Verification items for the finished model (mm, model axes). A direction names the side the tool comes from. Round coordinates to 2 decimals unless told otherwise and drop trailing zeros. Write each loop counter-clockwise with the first axis right and the second up, starting at its lowest first coordinate (ties: lowest second). Pieces come first, ordered by that corner, then holes. Notation, with made-up numbers: (-15.5, 2) - (38.5, 2) arc R35 ccw to (38.5, 37) - close; hole circle Ø8 at (-17.5, 78.25). An arc over 180 degrees is marked (long way). Answer as a JSON object with one key per item and string values. Group by question number.
1) Go/stop test with flat-tipped pins: pin 1 Ø2 at (x, z) = (-69, -39) entering from -Y; pin 2 Ø1.5 at (x, y) = (-13.5, 28.5) entering from -Z; pin 3 Ø4 at (x, y) = (-69.088, -30.988) entering from -Z. Record where each tip stops, or that it passes through.
2) Set-up check for faces 3 (the flat face through (1, 44.45, -47)), 4 (the cylindrical face through (-17.02, 21.68, 3.22)), 5 (the cylindrical face through (32.747, 47.669, -21.646)): record each of +Z, -Z, +X, -X, +Y, -Y from which the full face is reachable in a straight line by a thin tool's end or side.
3) Section check C-C (y = -1.5). Enter the section's corners in (x, z), then the cut area to 3 significant figures.
4) Section check A-A (x = 23.5). Enter the section's corners in (y, z) (3 decimals).
5) Mould release check, pull along Z, two halves, no side actions. Record for faces 1 (the cylindrical face through (32.747, 47.669, -59.746)), 2 (the cylindrical face through (66.568, 29.056, 3.131)): +Z half, -Z half, draft (parallel to the pull), parting line (faces both ways), or undercut.
6) Section check D-D (x = -75). Enter the section's corners in (y, z).
7) Section check B-B (z = -18.65). Enter the section's corners in (x, y) (3 decimals), then the cut area to 3 significant figures.
8) Thickness scan on line 1 (X direction, y = 48.75, z = -18.65) (3 decimals); line 2 (Y direction, x = -78, z = -62); line 3 (Z direction, x = 16, y = 22.5). Record the ranges inside material, lowest first.
```python
from build123d import *

# Parameters (mm, degrees)
SKETCH1_W           = 177.8
SKETCH1_H           = 101.6
SKETCH1_R           = 3.175
SKETCH1_W_2         = 46.99
SKETCH1_H_2         = 46.99
BOSS_EXTRUDE2_DEPTH = 6.35
SKETCH2_W           = 177.8
SKETCH2_H           = 6.35
BOSS_EXTRUDE3_DEPTH = 95.25
FILLET1_R           = 6.35
SKETCH3_R           = 4.065
CUT_EXTRUDE1_DEPTH  = 152.4


with BuildPart() as part:
    # Sketch1 → Boss-Extrude2 (new body)
    with BuildSketch(Plane.XY):
        Rectangle(SKETCH1_W, SKETCH1_H)
        with Locations((-69.088, 30.988)):
            Circle(SKETCH1_R, mode=Mode.SUBTRACT)
        with Locations((69.088, 30.988)):
            Circle(SKETCH1_R, mode=Mode.SUBTRACT)
        with Locations((69.088, -30.988)):
            Circle(SKETCH1_R, mode=Mode.SUBTRACT)
        with Locations((-69.088, -30.988)):
            Circle(SKETCH1_R, mode=Mode.SUBTRACT)
        with Locations((-38.608, 0)):
            Rectangle(SKETCH1_W_2, SKETCH1_H_2, mode=Mode.SUBTRACT)
        with Locations((38.608, 0)):
            Rectangle(SKETCH1_W_2, SKETCH1_H_2, mode=Mode.SUBTRACT)
    extrude(amount=BOSS_EXTRUDE2_DEPTH)

    # Sketch2 → Boss-Extrude3 (add)
    with BuildSketch(Plane(origin=(0, 0, 0), x_dir=(-1, 0, 0), z_dir=(0, 0, -1))):
        with Locations((0, 47.625)):
            Rectangle(SKETCH2_W, SKETCH2_H)
    extrude(amount=BOSS_EXTRUDE3_DEPTH)

    # Fillet1
    fillet1_edges = [part.edges().sort_by_distance(p)[0] for p in [
        (15.113, 23.495, 3.175),
        (15.113, -23.495, 3.175),
        (62.103, -23.495, 3.175),
        (62.103, 23.495, 3.175),
        (-62.103, 23.495, 3.175),
        (-62.103, -23.495, 3.175),
        (-15.113, -23.495, 3.175),
        (-15.113, 23.495, 3.175),
    ]]
    fillet(fillet1_edges, radius=FILLET1_R)

    # Sketch3 → Cut-Extrude1 (cut)
    with BuildSketch(Plane(origin=(0, 50.8, 0), x_dir=(1, 0, 0), z_dir=(0, 1, 0))):
        with Locations(Location((-30, 18.65, 0), (0, 0, 270))):
            Circle(SKETCH3_R)
        with Locations(Location((-30, 56.75, 0), (0, 0, 270))):
            Circle(SKETCH3_R)
        with Locations(Location((30, 18.65, 0), (0, 0, 270))):
            Circle(SKETCH3_R)
        with Locations(Location((30, 56.75, 0), (0, 0, 270))):
            Circle(SKETCH3_R)
    extrude(amount=-CUT_EXTRUDE1_DEPTH, mode=Mode.SUBTRACT)


solid = part.part
```
Returned:
{
 "1": {"pin 1": "y = 44.45", "pin 2": "z = 0", "pin 3": "through"},
 "2": {"face 3": "-Z, +X, -X, -Y", "face 4": "+Z, -Z", "face 5": "+Y, -Y"},
 "3": {"outline": "(-88.9, 0) - (-62.1, 0) - (-62.1, 6.35) - (-88.9, 6.35) - close; (-15.11, 0) - (15.11, 0) - (15.11, 6.35) - (-15.11, 6.35) - close; (62.1, 0) - (88.9, 0) - (88.9, 6.35) - (62.1, 6.35) - close", "area": "532 mm2"},
 "4": {"outline": "(-50.8, 0) - (-23.495, 0) - (-23.495, 6.35) - (-50.8, 6.35) - close; (23.495, 0) - (44.45, 0) - (44.45, -95.25) - (50.8, -95.25) - (50.8, 6.35) - (23.495, 6.35) - close"},
 "5": {"face 1": "undercut", "face 2": "draft"},
 "6": {"outline": "(-50.8, 0) - (44.45, 0) - (44.45, -95.25) - (50.8, -95.25) - (50.8, 6.35) - (-50.8, 6.35) - close"},
 "7": {"outline": "(-88.9, 44.45) - (-34.065, 44.45) - (-34.065, 50.8) - (-88.9, 50.8) - close; (-25.935, 44.45) - (25.935, 44.45) - (25.935, 50.8) - (-25.935, 50.8) - close; (34.065, 44.45) - (88.9, 44.45) - (88.9, 50.8) - (34.065, 50.8) - close", "area": "1,030 mm2"},
 "8": {"line 1": "-88.9 to -34.065, -25.935 to 25.935, 34.065 to 88.9", "line 2": "44.45 to 50.8", "line 3": "0 to 6.35"}
}
